Design review of the part built by this model. Coordinates are the model's own, in mm. Face numbers are marked on the shaded views. A direction names the side the tool comes from. Give positions to 0.01 mm unless a question says otherwise; leave off trailing zeros. Order: outer loops, then holes, each group sorted by start corner. A loop starts at its lowest first (then second) coordinate and runs counter-clockwise, first axis right, second up. Notation, with made-up numbers: (-4.75, -4) -> (3.25, -4) arc R23 ccw to (3.25, 22) -> close; hole circle Ø9 at (89.5, 77). An arc over 180 degrees is marked (long way). Return JSON: item names as keys, results as strings.
```python
from build123d import *

# Parameters (mm, degrees)
F0_R     = 4.35
F1_DEPTH = 0.6
F2_R     = 2.2
F3_DEPTH = 0.2
F4_R     = 1.575
F4_R_2   = 1.395
F5_DEPTH = 0.95
F6_R     = 0.3


with BuildPart() as f1:
    # F0 (on Top) → F1 (new body)
    with BuildSketch(Plane.XY):
        Circle(F0_R)
    extrude(amount=F1_DEPTH)

    # F2 (on face) → F3 (join)
    with BuildSketch(Plane.XY.offset(0.6)):
        Circle(F2_R)
    extrude(amount=F3_DEPTH)

    # F4 (on face) → F5 (join)
    with BuildSketch(Plane.XY.offset(0.8)):
        Circle(F4_R)
        Circle(F4_R_2, mode=Mode.SUBTRACT)
    extrude(amount=F5_DEPTH)

    # F6
    f6_edges = [f1.edges().sort_by_distance(p)[0] for p in [
        (-4.35, 0, 0.6),
    ]]
    fillet(f6_edges, radius=F6_R)


solid = f1.part
```
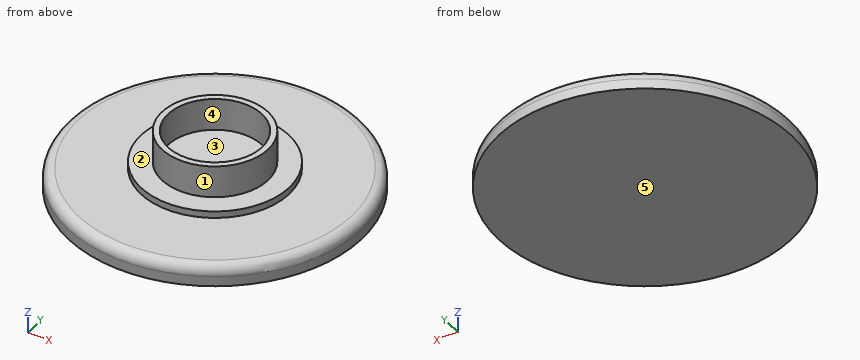
Item 1: For pin 1 (2 mm diameter, centred on x = 0, y = 0, fed in from -Z); pin 2 (1 mm diameter, centred on x = -2, y = 1, fed in from +Z), all flat-tipped, find the tip position at first contact; note any pin that passes through.
Result set:
{"pin 1": "stops at z = 0", "pin 2": "stops at z = 0.8"}
Item 2: Add section A-A (x = 0). Give the boundary of the cut face in (y, z) (3 decimals), plus the area to 3 significant figures.
Result set:
{"outline": "(-4.35, 0) -> (4.35, 0) -> (4.35, 0.3) arc R0.3 ccw to (4.05, 0.6) -> (2.2, 0.6) -> (2.2, 0.8) -> (1.575, 0.8) -> (1.575, 1.75) -> (1.395, 1.75) -> (1.395, 0.8) -> (-1.395, 0.8) -> (-1.395, 1.75) -> (-1.575, 1.75) -> (-1.575, 0.8) -> (-2.2, 0.8) -> (-2.2, 0.6) -> (-4.05, 0.6) arc R0.3 ccw to (-4.35, 0.3) -> close", "area": "6.40 mm^2"}
Item 3: Mouldability with a two-part tool opening along Y and no side actions: class the marked faces 1, 2 and 3 as released by +Y, released by -Y, zero draft, split by the parting line, or undercut.
Result set:
{"face 1": "split by the parting line", "face 2": "zero draft", "face 3": "undercut"}
Item 4: Add section B-B (z = 1.4). Give the boundary of the cut face in (x, y) (3 decimals).
Result set:
{"outline": "circle Ø3.15 at (0, 0); hole circle Ø2.79 at (0, 0)"}
Item 5: Machinability: for the marked faces 4 and 5, which of the approach directions +Z, -Z, +X, -X, +Y, -Y give a long, thin tool a straight path to every point of the face, cutting with its end or side? Answer none if there is none.
Result set:
{"face 4": "+Z", "face 5": "-Z, +X, -X, +Y, -Y"}
Item 6: Add section C-C (z = 0.5). Give the boundary of the cut face in (x, y), plus the area to 3 significant figures.
Result set:
{"outline": "circle Ø8.55 at (0, 0)", "area": "57.4 mm^2"}
Item 7: Wall thickness on L1, parallel to Y at x = 0, z = 1.4 (3 decimals); L2, parallel to Z at x = 3.5, y = -1; L3, parallel to Z at x = 0.75, y = 0.5: over which ranges is each line inside the solid? List them lowest first. Write a range as [from, to].
Result set:
{"L1": "y = [-1.575, -1.395], [1.395, 1.575]", "L2": "z = [0, 0.6]", "L3": "z = [0, 0.8]"}
